Here's how the part is built. I have some questions about the finished solid (model axes, mm). A direction names the side the tool comes from. Round coordinates to 2 decimals unless told otherwise and drop trailing zeros. Order: outer loops, then holes, each group sorted by start corner. A loop starts at its lowest first (then second) coordinate and runs counter-clockwise, first axis right, second up. Notation, with made-up numbers: (80.25, -22) -> (92.25, -22) arc R15 ccw to (92.25, 1) -> close; hole circle Ø11 at (35.5, 12). An arc over 180 degrees is marked (long way). Answer in a Markdown table with one row per item.
```python
from build123d import *

# Parameters (mm, degrees)
CROQUIS2_W                                           = 50
CROQUIS2_H                                           = 50
CROQUIS2_R                                           = 3.5
SALIENTE_EXTRUIR2_DEPTH                              = 20
CROQUIS3_R                                           = 7.5
CORTAR_EXTRUIR1_DEPTH                                = 3
SALIENTE_EXTRUIR3_DEPTH                              = 40
SALIENTE_EXTRUIR4_DEPTH                              = 2.65
CORTAR_EXTRUIR2_START                                = -2
CORTAR_EXTRUIR2_DEPTH                                = 5
SALIENTE_EXTRUIR5_START                              = -20.5
SALIENTE_EXTRUIR5_DEPTH                              = 13
SALIENTE_EXTRUIR6_START                              = -5
SALIENTE_EXTRUIR6_DEPTH                              = 3
REDONDEO1_R                                          = 2
CROQUIS12_R                                          = 2
CORTAR_EXTRUIR4_DEPTH                                = 2
CROQUIS13_R                                          = 2
CORTAR_EXTRUIR5_DEPTH                                = 3
REFRENTADO_PARA_TORNILLO_TAP_N_CON_CABEZ_D           = 4.5
REFRENTADO_PARA_TORNILLO_TAP_N_CON_CABEZ_CSINK_D     = 8.96
REFRENTADO_PARA_TORNILLO_TAP_N_CON_CABEZ_CSINK_ANGLE = 90
REDONDEO1_OF_SIMETR_A4_R                             = 2


with BuildPart() as part:
    # Croquis2 → Saliente-Extruir2 (new body)
    with BuildSketch(Plane.XY):
        Rectangle(CROQUIS2_W, CROQUIS2_H)
        Circle(CROQUIS2_R, mode=Mode.SUBTRACT)
    extrude(amount=SALIENTE_EXTRUIR2_DEPTH)

    # Croquis3 → Cortar-Extruir1 (cut)
    with BuildSketch(Plane.XY.offset(20)):
        Circle(CROQUIS3_R)
    extrude(amount=-CORTAR_EXTRUIR1_DEPTH, mode=Mode.SUBTRACT)

    # Croquis4 → Saliente-Extruir3 (add)
    with BuildSketch(Plane(origin=(0, 0, 0), x_dir=(-1, 0, 0), z_dir=(0, 0, -1))):
        Polygon((-25, -25), (-25, 17.4), (-28, 17.4), (-28, -28), (17.4, -28), (17.4, -25), align=None)
    extrude(amount=-SALIENTE_EXTRUIR3_DEPTH)

    # Croquis5 → Saliente-Extruir4 (add)
    with BuildSketch(Plane(origin=(0, 17.4, 0), x_dir=(1, 0, 0), z_dir=(0, 1, 0))):
        Polygon((25, 0), (51, 0), (26, -25), (25, -25), align=None)
    saliente_extruir4 = extrude(amount=-SALIENTE_EXTRUIR4_DEPTH)

    # Croquis6 → Cortar-Extruir2 (cut)
    with BuildSketch(Plane.XZ.offset(-14.75).offset(CORTAR_EXTRUIR2_START)):
        Polygon((44.915346148, 4.67044029), (30.667144507, 18.918641931), (26.318437803, 14.569935226), (40.566639444, 0.321733585), align=None)
    cortar_extruir2 = extrude(amount=CORTAR_EXTRUIR2_DEPTH, mode=Mode.SUBTRACT)

    # Simetría2: Saliente-Extruir4, Cortar-Extruir2 across plane
    add(saliente_extruir4.mirror(Plane(origin=(0, 0, 0), x_dir=(0, 0, 1), z_dir=(0.707106781, 0.707106781, 0))))
    add(cortar_extruir2.mirror(Plane(origin=(0, 0, 0), x_dir=(0, 0, 1), z_dir=(0.707106781, 0.707106781, 0))), mode=Mode.SUBTRACT)

    # Croquis10 → Saliente-Extruir5 (add)
    with BuildSketch(Plane.XZ.offset(28).offset(SALIENTE_EXTRUIR5_START)):
        Polygon((28, 0), (78, 0), (89, 0), (89, 2), (76, 2), (28, 50), (28, 61), (25, 61), (25, 40), (28, 40), align=None)
        Polygon((30, 45.171572875), (73.171572875, 2), (30, 2), align=None, mode=Mode.SUBTRACT)
    saliente_extruir5 = extrude(amount=-SALIENTE_EXTRUIR5_DEPTH)

    # Croquis11 → Saliente-Extruir6 (add)
    with BuildSketch(Plane.XZ.offset(7.5).offset(SALIENTE_EXTRUIR6_START)):
        Polygon((30, 45.171572875), (30, 2), (73.171572875, 2), align=None)
        Polygon((32, 40.343145751), (32, 4), (68.343145751, 4), align=None, mode=Mode.SUBTRACT)
    saliente_extruir6 = extrude(amount=-SALIENTE_EXTRUIR6_DEPTH)

    # Redondeo1
    redondeo1_edges = [part.edges().sort_by_distance(p)[0] for p in [
        (68.343145751, -1, 4),
        (32, -1, 4),
        (32, -1, 40.343145751),
    ]]
    fillet(redondeo1_edges, radius=REDONDEO1_R)

    # Croquis12 → Cortar-Extruir4 (cut)
    with BuildSketch(Plane.XY.offset(2)):
        with Locations((82.5, -1)):
            Circle(CROQUIS12_R)
    cortar_extruir4 = extrude(amount=-CORTAR_EXTRUIR4_DEPTH, mode=Mode.SUBTRACT)

    # Croquis13 → Cortar-Extruir5 (cut)
    with BuildSketch(Plane(origin=(28, 0, 0), x_dir=(0, 0, -1), z_dir=(1, 0, 0))):
        with Locations((-55.5, -1)):
            Circle(CROQUIS13_R)
    cortar_extruir5 = extrude(amount=-CORTAR_EXTRUIR5_DEPTH, mode=Mode.SUBTRACT)

    # Refrentado para tornillo tap_n con cabez (through all)
    with Locations(Plane(origin=(28, 0, 0), x_dir=(0, 0, -1), z_dir=(1, 0, 0))):
        with Locations((-55.5, -1)):
            refrentado_para_tornillo_tap_n_con_cabez = CounterSinkHole(REFRENTADO_PARA_TORNILLO_TAP_N_CON_CABEZ_D / 2, REFRENTADO_PARA_TORNILLO_TAP_N_CON_CABEZ_CSINK_D / 2, counter_sink_angle=REFRENTADO_PARA_TORNILLO_TAP_N_CON_CABEZ_CSINK_ANGLE)

    # Croquis17 → Refrentado para tornillo tap_n con c 2 (revolve, cut)
    with BuildSketch(Plane(origin=(82.5, -1, 2), x_dir=(0, -1, 0), z_dir=(1, 0, 0))):
        Polygon((0, 0), (0, 2), (2.25, 2), (2.25, 2.23), (4.48, 0), align=None)
    refrentado_para_tornillo_tap_n_con_c_2 = revolve(axis=Axis((82.5, -1, 8.35), (0, 0, -1)), mode=Mode.SUBTRACT)

    # Simetría4: Saliente-Extruir5, Saliente-Extruir6, Cortar-Extruir4, Cortar-Extruir5, Refrentado para tornillo tap_n con cabez, Refrentado para tornillo tap_n con c 2 across plane
    add(saliente_extruir5.mirror(Plane(origin=(0, 0, 0), x_dir=(0, 0, 1), z_dir=(0.707106781, 0.707106781, 0))))
    add(saliente_extruir6.mirror(Plane(origin=(0, 0, 0), x_dir=(0, 0, 1), z_dir=(0.707106781, 0.707106781, 0))))
    add(cortar_extruir4.mirror(Plane(origin=(0, 0, 0), x_dir=(0, 0, 1), z_dir=(0.707106781, 0.707106781, 0))), mode=Mode.SUBTRACT)
    add(cortar_extruir5.mirror(Plane(origin=(0, 0, 0), x_dir=(0, 0, 1), z_dir=(0.707106781, 0.707106781, 0))), mode=Mode.SUBTRACT)
    add(refrentado_para_tornillo_tap_n_con_cabez.mirror(Plane(origin=(0, 0, 0), x_dir=(0, 0, 1), z_dir=(0.707106781, 0.707106781, 0))), mode=Mode.SUBTRACT)
    add(refrentado_para_tornillo_tap_n_con_c_2.mirror(Plane(origin=(0, 0, 0), x_dir=(0, 0, 1), z_dir=(0.707106781, 0.707106781, 0))), mode=Mode.SUBTRACT)

    # Redondeo1 of Simetría4
    redondeo1_of_simetr_a4_edges = [part.edges().sort_by_distance(p)[0] for p in [
        (1, -68.343145751, 4),
        (1, -32, 4),
        (1, -32, 40.343145751),
    ]]
    fillet(redondeo1_of_simetr_a4_edges, radius=REDONDEO1_OF_SIMETR_A4_R)


solid = part.part
```
1. For faces 1 (the face through (-15.4, -33.34, 7.55)), 2 (the face through (-14.75, -35, 5)), 3 (the face through (-2.97, -51.28, 23.89)), which set-ups out of +Z, -Z, +X, -X, +Y, -Y let a thin tool reach every point of the face, with its end or its side?
Numbers:
| item | result |
|---|---|
| face 1 | none |
| face 2 | +Z, -Z, -Y |
| face 3 | -X |
2. Suppose I cut it at B-B on x = 82.5. Write out the boundary of the cut face in (y, z).
Numbers:
| item | result |
|---|---|
| outline | (-7.5, 0) -> (-3.48, 0) -> (-5.48, 2) -> (-7.5, 2) -> close; (1.48, 0) -> (5.5, 0) -> (5.5, 2) -> (3.48, 2) -> close |
3. Suppose I cut it at C-C on y = -82.5. Write out the boundary of the cut face in (x, z).
Numbers:
| item | result |
|---|---|
| outline | (-5.5, 0) -> (-1.48, 0) -> (-3.48, 2) -> (-5.5, 2) -> close; (3.48, 0) -> (7.5, 0) -> (7.5, 2) -> (5.48, 2) -> close |
4. Please list where these lines run through material, in increasing order: line 1 along Y through (x, z) = (25.4, 55.5); line 2 along X through (y, z) = (0, 10.75); line 3 along Y through (x, z) = (11, 26).
Numbers:
| item | result |
|---|---|
| line 1 | y = -7.5 to -3.25, 1.25 to 5.5 |
| line 2 | x = -25 to -3.5, 3.5 to 32, 61.59 to 67.25 |
| line 3 | y = -28 to -25 |
5. Suppose I cut it at D-D on z = 42.5. Write out the boundary of the cut face in (x, y), then the cut area to 3 significant figures.
Numbers:
| item | result |
|---|---|
| outline | (-5.5, -35.5) -> (7.5, -35.5) -> (7.5, -32.67) -> (2.5, -32.67) -> (2.5, -30) -> (7.5, -30) -> (7.5, -25) -> (-5.5, -25) -> (-5.5, -30) -> (-0.5, -30) -> (-0.5, -32.67) -> (-5.5, -32.67) -> close; (25, -7.5) -> (30, -7.5) -> (30, -2.5) -> (32.67, -2.5) -> (32.67, -7.5) -> (35.5, -7.5) -> (35.5, 5.5) -> (32.67, 5.5) -> (32.67, 0.5) -> (30, 0.5) -> (30, 5.5) -> (25, 5.5) -> close |
| area | 220 mm2 |
6. For pin 1 Ø11.5 at (y, z) = (-35, 10.5) entering from +X; pin 2 Ø4 at (y, z) = (1.5, 37) entering from -X; pin 3 Ø6 at (y, z) = (-15.5, 27.5) entering from +X, each with a flat end and sliding along its axis, tell me the tip position at first contact or that it passes through.
Numbers:
| item | result |
|---|---|
| pin 1 | stops at x = 7.5 |
| pin 2 | stops at x = 25 |
| pin 3 | stops at x = 28 |
7. We'd pull the mould along Y, two halves only. Please class faces 4 (the face through (84, -5.4, 2)), 5 (the face through (-21, -25, 10)), 6 (the face through (-15.4, -28.04, 16.29)): released by +Y, released by -Y, zero draft, split by the parting line, or undercut.
Numbers:
| item | result |
|---|---|
| face 4 | zero draft |
| face 5 | released by -Y |
| face 6 | undercut |
8. Suppose I cut it at A-A on z = 55.5. Write out the boundary of the cut face in (x, y), then the cut area to 3 significant figures.
Numbers:
| item | result |
|---|---|
| outline | (-5.5, -28) -> (-3.48, -28) -> (-1.25, -25.77) -> (-1.25, -25) -> (-5.5, -25) -> close; (3.25, -25.77) -> (5.48, -28) -> (7.5, -28) -> (7.5, -25) -> (3.25, -25) -> close; (25, -7.5) -> (28, -7.5) -> (28, -5.48) -> (25.77, -3.25) -> (25, -3.25) -> close; (25, 1.25) -> (25.77, 1.25) -> (28, 3.48) -> (28, 5.5) -> (25, 5.5) -> close |
| area | 41.1 mm2 |
